For this review, take the finished solid that the model builds, in its own axes (mm). A direction names the side the tool comes from. Give positions to 0.01 mm unless a question says otherwise; leave off trailing zeros. Loops run counter-clockwise (first coordinate to the right, second up) from the corner with the lowest first, then second, coordinate; pieces in that order, holes last.
```python
from build123d import *

# Parameters (mm, degrees)
BOSS_EXTRUDE1_DEPTH = 9
SKETCH4_W           = 67
SKETCH4_H           = 29
CUT_EXTRUDE1_DEPTH  = 4
SKETCH7_W           = 27
SKETCH7_H           = 2.5
CUT_EXTRUDE2_DEPTH  = 19
SKETCH9_W           = 57
SKETCH9_H           = 29
CUT_EXTRUDE3_DEPTH  = 4
SKETCH10_W          = 16
SKETCH10_H          = 3
CUT_EXTRUDE4_DEPTH  = 4
BOSS_EXTRUDE4_DEPTH = 10


with BuildPart() as part:
    # Sketch1 → Boss-Extrude1 (new body)
    with BuildSketch(Plane(origin=(0, 0, 0), x_dir=(1, 0, 0), z_dir=(0, 1, 0))):
        with BuildLine():
            Line((-32.5, -15.5), (32.5, -15.5))
            ThreePointArc((32.5, -15.5), (33.914213562, -14.914213562), (34.5, -13.5))
            Line((34.5, -13.5), (34.5, 13.5))
            ThreePointArc((34.5, 13.5), (33.914213562, 14.914213562), (32.5, 15.5))
            Line((32.5, 15.5), (-32.5, 15.5))
            ThreePointArc((-32.5, 15.5), (-33.914213562, 14.914213562), (-34.5, 13.5))
            Line((-34.5, 13.5), (-34.5, -13.5))
            ThreePointArc((-34.5, -13.5), (-33.914213562, -14.914213562), (-32.5, -15.5))
        make_face()
    extrude(amount=BOSS_EXTRUDE1_DEPTH)

    # Sketch4 → Cut-Extrude1 (cut)
    with BuildSketch(Plane(origin=(0, 9, 0), x_dir=(1, 0, 0), z_dir=(0, 1, 0))):
        Rectangle(SKETCH4_W, SKETCH4_H)
    extrude(amount=-CUT_EXTRUDE1_DEPTH, mode=Mode.SUBTRACT)

    # Sketch7 → Cut-Extrude2 (cut)
    with BuildSketch(Plane.ZY.offset(-33.5)):
        with Locations((0, 7.75)):
            Rectangle(SKETCH7_W, SKETCH7_H)
    extrude(amount=-CUT_EXTRUDE2_DEPTH, mode=Mode.SUBTRACT)

    # Sketch9 → Cut-Extrude3 (cut)
    with BuildSketch(Plane(origin=(0, 5, 0), x_dir=(1, 0, 0), z_dir=(0, 1, 0))):
        Rectangle(SKETCH9_W, SKETCH9_H)
    extrude(amount=-CUT_EXTRUDE3_DEPTH, mode=Mode.SUBTRACT)

    # Sketch10 → Cut-Extrude4 (cut)
    with BuildSketch(Plane(origin=(-33.5, 0, 0), x_dir=(0, 0, -1), z_dir=(1, 0, 0))):
        with Locations((0, 7.5)):
            Rectangle(SKETCH10_W, SKETCH10_H)
    extrude(amount=-CUT_EXTRUDE4_DEPTH, mode=Mode.SUBTRACT)

    # Sketch13 → Boss-Extrude4 (add, symmetric)
    with BuildSketch(Plane(origin=(0, 0, 0), x_dir=(0, 0, -1), z_dir=(1, 0, 0))):
        Polygon((14.5, 7), (14.5, 9), (13.75, 8), align=None)
        Polygon((-13.75, 8), (-14.5, 7), (-14.5, 9), align=None)
    extrude(amount=BOSS_EXTRUDE4_DEPTH, both=True)


solid = part.part
```
Item 1: Clearance check with flat-ended pins moving along their axes: pin 1 Ø1.5 at (x, z) = (30, 6.5) entering from +Y; pin 2 Ø0.8 at (x, z) = (-34, -2) entering from +Y; pin 3 Ø0.8 at (x, z) = (34, 1.5) entering from +Y; pin 4 Ø10 at (x, z) = (21, -9) entering from -Y. State where each tip first meets the part, or that it passes through.
Answer:
pin 1: stops at y = 5
pin 2: stops at y = 6
pin 3: stops at y = 6.5
pin 4: stops at y = 0
Item 2: Take a section at B-B on z = 11. Give the boundary of the cut face in (x, y).
Answer:
outline: (-34.5, 0) - (34.5, 0) - (34.5, 6.5) - (33.5, 6.5) - (33.5, 5) - (28.5, 5) - (28.5, 1) - (-28.5, 1) - (-28.5, 5) - (-33.5, 5) - (-33.5, 9) - (-34.5, 9) - close
Item 3: Tool access review of faces 1 (the flat face through (0, 4, 15.5)), 2 (the flat face through (28.5, 3, 0)), 3 (the flat face through (0, 5, -14.5)): name each direction out of +Z, -Z, +X, -X, +Y, -Y from which nothing blocks a thin tool from reaching the whole face with its end or side.
Answer:
face 1: +Z, +X, -X, +Y, -Y
face 2: +Y
face 3: none
Item 4: For L1, parallel to Z at x = -30.5, y = 5.75; L2, parallel to X at y = 1.25, z = -1; L3, parallel to Y at x = 2.5, z = -6.5, list the stretches that pass through material, from the lowest coordinate up.
Answer:
L1: z = -15.5 to -14.5, 14.5 to 15.5
L2: x = -34.5 to -28.5, 28.5 to 34.5
L3: y = 0 to 1
Item 5: Take a section at D-D on z = 0. Give the boundary of the cut face in (x, y).
Answer:
outline: (-34.5, 0) - (34.5, 0) - (34.5, 6.5) - (33.5, 6.5) - (33.5, 5) - (28.5, 5) - (28.5, 1) - (-28.5, 1) - (-28.5, 5) - (-33.5, 5) - (-33.5, 6) - (-34.5, 6) - close
Item 6: Take a section at A-A on y = 4. Give the boundary of the cut face in (x, z).
Answer:
outline: (-34.5, -13.5) arc R2 ccw to (-32.5, -15.5) - (32.5, -15.5) arc R2 ccw to (34.5, -13.5) - (34.5, 13.5) arc R2 ccw to (32.5, 15.5) - (-32.5, 15.5) arc R2 ccw to (-34.5, 13.5) - close; hole (-28.5, -14.5) - (28.5, -14.5) - (28.5, 14.5) - (-28.5, 14.5) - close
Item 7: The part is to be moulded in two halves that separate along Z. For faces 4 (the cylindrical face through (-33.9, 4.44, -14.93)), 5 (the flat face through (34.5, 3, 0)), 6 (the cylindrical face through (33.9, 4.44, 14.93)), 7 (the flat face through (33.5, 6, 0)), say which applies: released by +Z, released by -Z, zero draft, split by the parting line, or undercut.
Answer:
face 4: released by -Z
face 5: zero draft
face 6: released by +Z
face 7: undercut
Item 8: Take a section at C-C on x = -15.5. Give the boundary of the cut face in (y, z).
Answer:
outline: (0, -15.5) - (9, -15.5) - (9, -14.5) - (1, -14.5) - (1, 14.5) - (9, 14.5) - (9, 15.5) - (0, 15.5) - close
